The model under review builds one solid part; all positions refer to its coordinate system, in mm. A direction names the side the tool comes from. Round coordinates to 2 decimals unless told otherwise and drop trailing zeros. Loops run counter-clockwise (first coordinate to the right, second up) from the corner with the lowest first, then second, coordinate; pieces in that order, holes last. Notation, with made-up numbers: (42, -34) -> (84, -34) arc R15 ccw to (84, -16) -> close; hole circle Ø10 at (22, 24). An arc over 180 degrees is marked (long way). Return JSON: item names as keys, results as strings. Group by question number.
```python
from build123d import *

# Parameters (mm, degrees)
BOSS_EXTRUDE1_DEPTH  = 6.35
M4_CLEARANCE_HOLE1_D = 4.5
FILLET1_R            = 1.905


with BuildPart() as part:
    # Sketch1 → Boss-Extrude1 (new body)
    with BuildSketch(Plane.XY):
        with BuildLine():
            Line((0, 0), (-12.7, 0))
            ThreePointArc((-12.7, 0), (-24.638, 11.938), (-36.576, 0))
            Line((-36.576, 0), (-49.276, 0))
            Line((-49.276, 0), (-49.276, 4.318))
            Line((-49.276, 4.318), (-39.116, 4.318))
            ThreePointArc((-39.116, 4.318), (-24.638, 13.627054389), (-10.16, 4.318))
            Line((-10.16, 4.318), (0, 4.318))
            Line((0, 4.318), (0, 0))
        make_face()
    extrude(amount=BOSS_EXTRUDE1_DEPTH)

    # M4 Clearance Hole1 (through all)
    with Locations(Plane(origin=(0, 4.318, 0), x_dir=(1, 0, 0), z_dir=(0, 1, 0))):
        with Locations((-4.1275, -3.175)):
            m4_clearance_hole1 = Hole(M4_CLEARANCE_HOLE1_D / 2)

    # Fillet1
    fillet1_edges = [part.edges().sort_by_distance(p)[0] for p in [
        (-39.116, 4.318, 3.175),
        (-10.16, 4.318, 3.175),
    ]]
    fillet(fillet1_edges, radius=FILLET1_R)

    # Mirror1: M4 Clearance Hole1 across plane
    add(m4_clearance_hole1.mirror(Plane(origin=(-24.638, 0, 0), x_dir=(0, 0, 1), z_dir=(1, 0, 0))), mode=Mode.SUBTRACT)


solid = part.part
```
1. We need section B-B, the plane z = 4.5. Write out the cut boundary in (x, y) (3 decimals), then the cut area to 3 significant figures.
2. We need section C-C, the plane x = -3.5. Write out the cut boundary in (y, z), then the cut area to 3 significant figures.
3. For P1, Ø3, axis at x = -44, z = 2, coming from the +Y side; P2, Ø1.5, axis at x = -25.5, z = 2, coming from the -Y side, all flat-tipped, find the tip position at first contact; note any pin that passes through.
4. Wall thickness on line 1 (X direction, y = 2.75, z = 2.5); line 2 (X direction, y = 2.75, z = 3.5); line 3 (X direction, y = 8, z = 5.5): over which ranges is each line inside the solid? List them lowest first.
5. We need section D-D, the plane z = 1.5. Write out the cut boundary in (x, y) (3 decimals).
6. We need section A-A, the plane y = 8. Write out the cut boundary in (x, z).
7. Draft analysis for pull direction X (two halves, no side actions). For faces 4 (the face through (0, 2, 3)), 5 (the face through (-24.375, 11.935, 3.131)), 6 (the face through (-41, 0, 3)), state which applies: pulls with the +X half, pulls with the -X half, needs draft (parallel to the pull), parting line crosses it, or undercut.
8. Tool access review of faces 1 (the face through (-7, 4.318, 3)), 2 (the face through (-43, 4.318, 2)), 3 (the face through (-8, 0, 3)): name each direction out of +Z, -Z, +X, -X, +Y, -Y from which nothing blocks a thin tool from reaching the whole face with its end or side.
Check sheet entries:
{
 "1": {"outline": "(-49.276, 0) -> (-46.967, 0) -> (-46.967, 4.318) -> (-49.276, 4.318) -> close; (-43.33, 0) -> (-36.576, 0) arc R11.938 cw to (-12.7, 0) -> (-5.946, 0) -> (-5.946, 4.318) -> (-8.983, 4.318) arc R1.905 cw to (-10.657, 5.313) arc R15.913 ccw to (-38.619, 5.313) arc R1.905 cw to (-40.293, 4.318) -> (-43.33, 4.318) -> close; (-2.309, 0) -> (0, 0) -> (0, 4.318) -> (-2.309, 4.318) -> close", "area": "152 mm²"},
 "2": {"outline": "(0, 0) -> (4.32, 0) -> (4.32, 1.01) -> (0, 1.01) -> close; (0, 5.34) -> (4.32, 5.34) -> (4.32, 6.35) -> (0, 6.35) -> close", "area": "8.76 mm²"},
 "3": {"P1": "stops at y = 4.32", "P2": "stops at y = 11.83"},
 "4": {"line 1": "x = -49.28 to -47.29, -43 to -36.25, -13.02 to -6.27, -1.98 to 0", "line 2": "x = -49.28 to -47.37, -42.92 to -36.25, -13.02 to -6.35, -1.9 to 0", "line 3": "x = -36.78 to -33.5, -15.78 to -12.5"},
 "5": {"outline": "(-49.276, 0) -> (-46.651, 0) -> (-46.651, 4.318) -> (-49.276, 4.318) -> close; (-43.646, 0) -> (-36.576, 0) arc R11.938 cw to (-12.7, 0) -> (-5.63, 0) -> (-5.63, 4.318) -> (-8.983, 4.318) arc R1.905 cw to (-10.657, 5.313) arc R15.913 ccw to (-38.619, 5.313) arc R1.905 cw to (-40.293, 4.318) -> (-43.646, 4.318) -> close; (-2.625, 0) -> (0, 0) -> (0, 4.318) -> (-2.625, 4.318) -> close"},
 "6": {"outline": "(-36.78, 0) -> (-33.5, 0) -> (-33.5, 6.35) -> (-36.78, 6.35) -> close; (-15.78, 0) -> (-12.5, 0) -> (-12.5, 6.35) -> (-15.78, 6.35) -> close"},
 "7": {"face 4": "pulls with the +X half", "face 5": "undercut", "face 6": "needs draft"},
 "8": {"face 1": "+Z, -Z, +X, +Y", "face 2": "+Z, -Z, -X, +Y", "face 3": "+Z, -Z, +X, -X, -Y"}
}
